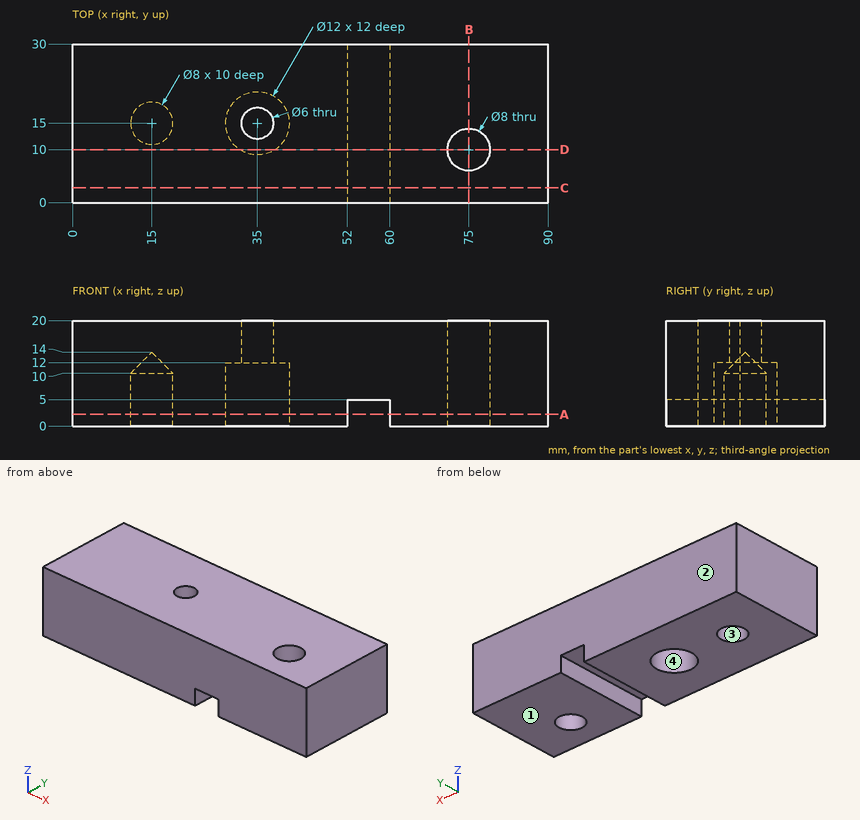
Study the drawing (mm; zero at the part's minimum x, y, z) and answer. Coordinates: 2 decimals unless noted, no trailing zeros. Loops run counter-clockwise (first coordinate to the right, second up) from the corner with the lowest first, then second, coordinate; pieces in that order, holes last. Notation, with made-up numbers: (51.25, 40) -> (87.25, 40) arc R8 ccw to (87.25, 51) -> close; hole circle Ø8 at (43.5, 71.25). An arc over 180 degrees is marked (long way). Write item = value, one per line. Start each with the question number.
1) The mould has two halves that part along Y. Classify the marked faces 1, 2, 3 and 4: pulls with the +Y half, pulls with the -Y half, needs draft (parallel to the pull), parting line crosses it, or undercut.
2) The part is cut by section A-A, the plane z = 2.25. Determine the outline of the cut face in (x, y).
3) Find the intervals of material crossed by L1, parallel to Y at x = 15, z = 2.25; L2, parallel to X at y = 16, z = 9.25; L3, parallel to Y at x = 35, z = 15.25, in increasing order. Write a range as from..to.
4) The part is cut by section B-B, the plane x = 75. Determine the outline of the cut face in (y, z), plus the area to 3 significant figures.
5) The part is cut by section C-C, the plane y = 2.75. Determine the outline of the cut face in (x, z), plus the area to 3 significant figures.
6) The part is cut by section D-D, the plane y = 10. Determine the outline of the cut face in (x, z), plus the area to 3 significant figures.
7) Given P1, Ø8, axis at x = 35, y = 15, coming from the -Z side; P2, Ø2.5, axis at x = 57.5, y = 22, coming from the -Z side, each flat-ended and moving along its own axis, determine where each tip first touches the part or whether it passes through.
Result:
q1.face_1 = needs draft
q1.face_2 = pulls with the +Y half
q1.face_3 = undercut
q1.face_4 = undercut
q2.outline = (0, 0) -> (52, 0) -> (52, 30) -> (0, 30) -> close; (60, 0) -> (90, 0) -> (90, 30) -> (60, 30) -> close; hole circle Ø8 at (15, 15); hole circle Ø12 at (35, 15); hole circle Ø8 at (75, 10)
q3.L1 = 0..11, 19..30
q3.L2 = 0..11.13, 18.87..29.08, 40.92..90
q3.L3 = 0..12, 18..30
q4.outline = (0, 0) -> (6, 0) -> (6, 20) -> (0, 20) -> close; (14, 0) -> (30, 0) -> (30, 20) -> (14, 20) -> close
q4.area = 440 mm²
q5.outline = (0, 0) -> (52, 0) -> (52, 5) -> (60, 5) -> (60, 0) -> (90, 0) -> (90, 20) -> (0, 20) -> close
q5.area = 1,760 mm²
q6.outline = (0, 0) -> (31.68, 0) -> (31.68, 12) -> (38.32, 12) -> (38.32, 0) -> (52, 0) -> (52, 5) -> (60, 5) -> (60, 0) -> (71, 0) -> (71, 20) -> (0, 20) -> close; (79, 0) -> (90, 0) -> (90, 20) -> (79, 20) -> close
q6.area = 1,520 mm²
q7.P1 = 12
q7.P2 = 5
